from build123d import *

# Parameters (mm, degrees)
BOSS_EXTRUDE1_DEPTH = 3
SKETCH2_W           = 30
SKETCH2_H           = 3
BOSS_EXTRUDE2_DEPTH = 27
BOSS_EXTRUDE3_DEPTH = 2
BOSS_EXTRUDE4_DEPTH = 2
CHAMFER1_SIZE       = 5
FILLET1_R           = 3


with BuildPart() as part:
    # Sketch1 → Boss-Extrude1 (new body)
    with BuildSketch(Plane(origin=(0, 0, 0), x_dir=(1, 0, 0), z_dir=(0, 1, 0))):
        Polygon((-5, 15), (15, 15), (15, -15), (-15, -15), (-15, 5), (-5, 5), align=None)
    extrude(amount=BOSS_EXTRUDE1_DEPTH)

    # Sketch2 → Boss-Extrude2 (add)
    with BuildSketch(Plane(origin=(0, 3, 0), x_dir=(1, 0, 0), z_dir=(0, 1, 0))):
        with Locations((0, -13.5)):
            Rectangle(SKETCH2_W, SKETCH2_H)
    extrude(amount=BOSS_EXTRUDE2_DEPTH)

    # Sketch3 → Boss-Extrude3 (add)
    with BuildSketch(Plane.ZY.offset(15)):
        Polygon((-5, 3), (12, 20), (12, 3), align=None)
    extrude(amount=-BOSS_EXTRUDE3_DEPTH)

    # Sketch4 → Boss-Extrude4 (add)
    with BuildSketch(Plane(origin=(15, 0, 0), x_dir=(0, 0, -1), z_dir=(1, 0, 0))):
        Polygon((-12, 20), (5, 3), (-12, 3), align=None)
    extrude(amount=-BOSS_EXTRUDE4_DEPTH)

    # Chamfer1
    chamfer1_edges = [part.edges().sort_by_distance(p)[0] for p in [
        (-15, 30, 13.5),
        (15, 30, 13.5),
    ]]
    chamfer(chamfer1_edges, length=CHAMFER1_SIZE)

    # Fillet1
    fillet1_edges = [part.edges().sort_by_distance(p)[0] for p in [
        (0, 3, 12),
    ]]
    fillet(fillet1_edges, radius=FILLET1_R)


solid = part.part
Verification items for the finished model (mm, model axes). A direction names the side the tool comes from. Coordinates: 2 decimals unless noted, no trailing zeros. Write each loop counter-clockwise with the first axis right and the second up, starting at its lowest first coordinate (ties: lowest second). Pieces come first, ordered by that corner, then holes. Notation, with made-up numbers: (-19.75, -15.5) -> (-14.75, -15.5) arc R13 cw to (-14.75, -4.5) -> close; hole circle Ø5 at (47.25, 23.25). An arc over 180 degrees is marked (long way). One line per item, written item: value. Start each with the question number.
Q1. Go/stop test with flat-tipped pins: P1, Ø1.5, axis at x = 6.5, y = 7, coming from the -Z side; P2, Ø1.5, axis at y = 2, z = -10, coming from the -X side; P3, Ø4, axis at x = 0.5, z = 8.5, coming from the +Y side. Record where each tip stops, or that it passes through.
Q2. Cross-section at A-A on y = 18.75. Enter the section's corners in (x, z).
Q3. Mould release check, pull along X, two halves, no side actions. Record for faces 1 (the flat face through (1, 3, -3)), 2 (the flat face through (-5, 1, -10)), 3 (the flat face through (15, 7, 6)): pulls with the +X half, pulls with the -X half, needs draft (parallel to the pull), parting line crosses it, or undercut.
Q4. Thickness scan on L1, parallel to X at y = 11, z = 5; L2, parallel to Y at x = 6.75, z = -6.25; L3, parallel to Z at x = -11.5, y = 18.75. Record the ranges inside material, lowest first. Write a range as from..to.
Q5. Cross-section at B-B on z = -0.25. Enter the section's corners in (x, y), and give its area (3 significant figures).
Q6. Cross-section at C-C on x = -10.5. Enter the section's corners in (y, z), and give its area (3 significant figures).
Q7. Access from +Z, -Z, +X, -X, +Y, -Y to the whole of each face (thin tool, end or side, straight path). Record for faces 4 (the flat face through (-10, 1, -5)), 5 (the flat face through (-13, 8, 7)), 6 (the flat face through (-13, 27, 14)).
Q8. Cross-section at D-D on x = -5.75. Enter the section's corners in (y, z), and give its area (3 significant figures).
Checked values:
1. P1: stops at z = 12
1. P2: stops at x = -5
1. P3: stops at y = 3.4
2. outline: (-15, 10.75) -> (-13, 10.75) -> (-13, 12) -> (13, 12) -> (13, 10.75) -> (15, 10.75) -> (15, 15) -> (-15, 15) -> close
3. face 1: undercut
3. face 2: pulls with the -X half
3. face 3: pulls with the +X half
4. L1: x = -15..-13, 13..15
4. L2: y = 0..3
4. L3: z = 12..15
5. outline: (-15, 0) -> (15, 0) -> (15, 7.75) -> (13, 7.75) -> (13, 3) -> (-13, 3) -> (-13, 7.75) -> (-15, 7.75) -> close
5. area: 109 mm²
6. outline: (0, -5) -> (3, -5) -> (3, 9) arc R3 cw to (6, 12) -> (29.5, 12) -> (29.5, 15) -> (0, 15) -> close
6. area: 141 mm²
7. face 4: -Z, -X, +Y, -Y
7. face 5: -Z, +Y
7. face 6: +Z, -Z, -X, +Y
8. outline: (0, -5) -> (3, -5) -> (3, 9) arc R3 cw to (6, 12) -> (30, 12) -> (30, 15) -> (0, 15) -> close
8. area: 143 mm²
